Geometry check sheet. Reference: the model listing, model coordinates, mm. A direction names the side the tool comes from. Round coordinates to 2 decimals unless told otherwise and drop trailing zeros. Order: outer loops, then holes, each group sorted by start corner. A loop starts at its lowest first (then second) coordinate and runs counter-clockwise, first axis right, second up. Notation, with made-up numbers: (37, -31) - (69, -31) arc R18 cw to (69, 2) - close; hole circle Ø2 at (3.5, 13). An arc over 180 degrees is marked (long way). Use a Markdown table: item, result. Add a question column.
(1) Mould release check, pull along Y, two halves, no side actions. Record for faces 3 (the face through (-48, -3.175, 2)), 4 (the face through (15.227, 0.625, 1.565)), 5 (the face through (3.16, -0.7, 1.61)), 6 (the face through (-79.489, 0, 2)): released by +Y, released by -Y, zero draft, split by the parting line, or undercut.
(2) Thickness scan on line 1 along X through (y, z) = (0, 1.15); line 2 along Y through (x, z) = (0, 1.35); line 3 along Y through (x, z) = (-18.5, 0.6) (3 decimals). Record the ranges inside material, lowest first. Write a range as [from, to].
(3) Access from +Z, -Z, +X, -X, +Y, -Y to the whole of each face (thin tool, end or side, straight path). Record for faces 1 (the face through (-12, 0, 3.175)), 2 (the face through (-47, 3.175, 2)).
(4) Section check B-B on y = 0. Record the boundary of the cut face in (x, z) (1 decimal).
(5) Section check A-A on x = 0. Record the boundary of the cut face in (y, z) (1 decimal).
(6) Section check C-C on z = 1.65. Record the boundary of the cut face in (x, y) (1 decimal), then the cut area to 3 significant figures.
(7) Gauge pin test, flat ends, axial feed: P1, Ø1.5, axis at x = -37, z = 1, coming from the -Y side (3 decimals); P2, Ø1.5, axis at x = -68.5, z = 2, coming from the +Y side (3 decimals). Record the tip position at first contact, or that the pin passes through.
(8) Section check D-D on x = -64.5. Record the boundary of the cut face in (y, z) (3 decimals).
Autodesk Inventor part; units mm, degrees
ref_plane "Work Plane1" through (-15.24, 0, 3.175) normal (1, 0, 0) x (0, 1, 0)
ref_plane "YZ Plane" through (0, 0, 0) normal (1, 0, 0) x (0, 1, 0)
ref_plane "XZ Plane" through (0, 0, 0) normal (0, 1, 0) x (-1, 0, 0)
sketch "Sketch1" plane through (0, 0, 0) normal (0, 0, 1) x (1, 0, 0)
  circle A0 centre (0, 0) radius 15.24
extrude "Extrusion1" add sketch "Sketch1" along normal blind 3.175
sketch "Sketch2" plane through (0, 0, 3.175) normal (0, 0, 1) x (1, 0, 0)
  circle A0 centre (0, 0) radius 15.24
  line L0 (-15.24, 0) -> (-15.24, 3.175)
  line L1 (-15.24, 0) -> (-15.24, -3.175)
  dimension "d3" = 3.175
  dimension "d4" = 3.175
ref_plane "Work Plane1" through (-15.24, 0, 3.175) normal (1, 0, 0) x (0, 1, 0)
sketch "Sketch3" plane through (-15.24, 0, 3.175) normal (1, 0, 0) x (0, 1, 0)
  line L0 (15.24, 0) -> (-15.24, 0)
  line L1 (-15.24, -3.175) -> (15.24, -3.175)
  line L2 (0, -3.175) -> (3.175, -3.175)
  line L3 (3.175, -3.175) -> (3.175, 0)
  line L4 (3.175, 0) -> (-3.175, 0)
  line L5 (-3.175, 0) -> (-3.175, -3.175)
  line L6 (-3.175, -3.175) -> (3.175, -3.175)
  dimension "d6" = 6.35
extrude "Extrusion2" add sketch "Sketch3" against normal blind 64.2493
sketch "Sketch4" plane through (-15.24, 0, 3.175) normal (1, 0, 0) x (0, 0, -1)
  line L0 (3.175, -3.175) -> (3.175, 0)
  line L1 (0, 3.175) -> (3.175, 3.175)
  line L2 (3.175, 3.175) -> (3.175, -3.175)
  line L3 (3.175, -3.175) -> (0, -3.175)
  line L4 (0, -3.175) -> (0, 3.175)
extrude "Extrusion3" add sketch "Sketch4" along normal blind 12.7
sketch "Sketch6" plane through (0, 0, 0) normal (0, 0, -1) x (-1, 0, 0)
  circle A0 centre (0, 0) radius 3.2385
  dimension "d24" = 6.477
hole "Hole1" at (0, 0, 0) direction (0, 0, -1) diameter 6.477 end through all
hole "Hole2" at (0, 0, 0) direction (0, 0, 1) diameter 6.477 depth 7.9375 tip angle 118
sketch "Sketch7" plane through (0, 0, 3.175) normal (0, 0, 1) x (1, 0, 0)
  line L0 (-79.4893, -3.175) -> (-79.4893, 3.175)
  line L1 (-79.4893, 0) -> (-76.3143, 0)
  circle A0 centre (-76.3143, 0) radius 1.5875
  point P0 (0, 0)
  dimension "d39" = 3.175
  dimension "d40" = 3.175
extrude "Extrusion6" cut sketch "Sketch7" against normal blind 25.4
properties part number "ClawLinkage"
Check sheet entries:
| question | item | result |
|---|---|---|
| 1 | face 3 | released by -Y |
| 1 | face 4 | split by the parting line |
| 1 | face 5 | undercut |
| 1 | face 6 | zero draft |
| 2 | line 1 | x = [-79.49, -77.9], [-74.73, -3.24], [3.24, 15.24] |
| 2 | line 2 | y = [-15.24, -3.24], [3.24, 15.24] |
| 2 | line 3 | y = [-3.175, 3.175] |
| 3 | face 1 | +Z, +X, -X, +Y, -Y |
| 3 | face 2 | +Z, -Z, -X, +Y |
| 4 | outline | (-79.5, 0) - (-77.9, 0) - (-77.9, 3.2) - (-79.5, 3.2) - close; (-74.7, 0) - (-3.2, 0) - (-3.2, 3.2) - (-74.7, 3.2) - close; (3.2, 0) - (15.2, 0) - (15.2, 3.2) - (3.2, 3.2) - close |
| 5 | outline | (-15.2, 0) - (-3.2, 0) - (-3.2, 3.2) - (-15.2, 3.2) - close; (3.2, 0) - (15.2, 0) - (15.2, 3.2) - (3.2, 3.2) - close |
| 6 | outline | (-79.5, -3.2) - (-14.9, -3.2) arc R15.2 ccw (long way) to (-14.9, 3.2) - (-79.5, 3.2) - close; hole circle Ø3.2 at (-76.3, 0); hole circle Ø6.5 at (0, 0) |
| 6 | area | 1,100 mm2 |
| 7 | P1 | stops at y = -3.175 |
| 7 | P2 | stops at y = 3.175 |
| 8 | outline | (-3.175, 0) - (3.175, 0) - (3.175, 3.175) - (-3.175, 3.175) - close |
